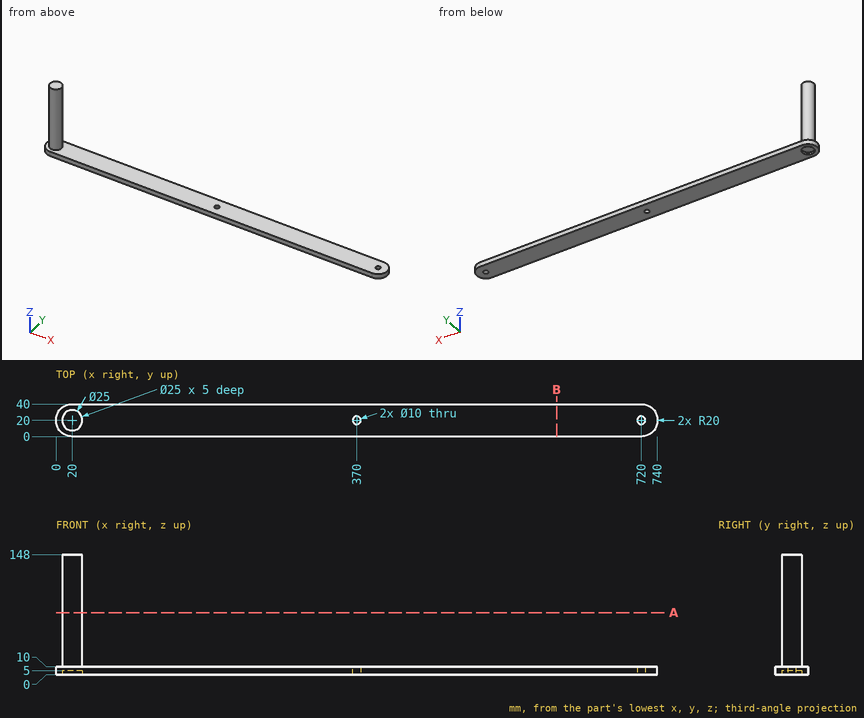
Design review of the part shown in the three views and the two pictorial views. Dimensions are in mm from the part's minimum x, y and z. Coordinates: 2 decimals unless noted, no trailing zeros. Write each loop counter-clockwise with the first axis right and the second up, starting at its lowest first coordinate (ties: lowest second). Pieces come first, ordered by that corner, then holes.
1) We need section B-B on x = 616. State the section outline as (y, z) points, then the cut area to 3 significant figures.
2) To check wall thickness, follow probe 1 along Y at (x, z) = (20, 3); probe 2 along Y at (x, z) = (720, 3); probe 3 along Z at (x, y) = (666, 17.5). State the ranges of each line that lie inside material, in increasing order.
3) Clearance check with flat-ended pins moving along their axes: pin 1 Ø12.5 at (x, y) = (24.5, 23.5) entering from -Z; pin 2 Ø20 at (x, y) = (222, 18) entering from +Z. State where each tip first meets the part, or that it passes through.
4) We need section A-A on z = 76.5. State the section outline as (x, y) points.
Answer list:
1. outline: (0, 0) - (40, 0) - (40, 10) - (0, 10) - close
1. area: 400 mm2
2. probe 1: y = 0 to 7.5, 32.5 to 40
2. probe 2: y = 0 to 15, 25 to 40
2. probe 3: z = 0 to 10
3. pin 1: stops at z = 5
3. pin 2: stops at z = 10
4. outline: circle Ø25 at (20, 20)
